from build123d import *

# Parameters (mm, degrees)
SKETCH1_R           = 1.05
BOSS_EXTRUDE1_DEPTH = 2.85
FILLET2_R           = 1
FILLET1_R           = 1


with BuildPart() as part:
    # Sketch1 → Boss-Extrude1 (new body)
    with BuildSketch(Plane.XY):
        with BuildLine():
            Line((2.236067977, 2), (15, 3.5))
            Line((15, 3.5), (15, 6))
            ThreePointArc((15, 6), (16.630733614, 7.494292047), (17.97721163, 5.739527733))
            Line((17.97721163, 5.739527733), (17.229668505, 1.5))
            Line((17.229668505, 1.5), (0, -2))
            Line((0, -2), (-17.229668505, 1.5))
            Line((-17.229668505, 1.5), (-17.97721163, 5.739527733))
            ThreePointArc((-17.97721163, 5.739527733), (-16.630733614, 7.494292047), (-15, 6))
            Line((-15, 6), (-15, 3.5))
            Line((-15, 3.5), (-2.236067977, 2))
            ThreePointArc((-2.236067977, 2), (0, 3), (2.236067977, 2))
        make_face()
        Circle(SKETCH1_R, mode=Mode.SUBTRACT)
    extrude(amount=BOSS_EXTRUDE1_DEPTH)

    # Fillet2
    fillet2_edges = [part.edges().sort_by_distance(p)[0] for p in [
        (15, 3.5, 1.425),
        (-15, 3.5, 1.425),
    ]]
    fillet(fillet2_edges, radius=FILLET2_R)

    # Fillet1
    fillet1_edges = [part.edges().sort_by_distance(p)[0] for p in [
        (15, 5.194681496, 0),
        (16.630733614, 7.494292047, 0),
        (17.603440067, 3.619763867, 0),
        (-17.603440067, 3.619763867, 0),
        (-16.630733614, 7.494292047, 0),
        (-16.630733614, 7.494292047, 2.85),
        (-8.176391715, 2.698098798, 0),
        (-17.603440067, 3.619763867, 2.85),
        (17.603440067, 3.619763867, 2.85),
        (16.630733614, 7.494292047, 2.85),
        (15, 5.194681496, 2.85),
        (-15, 5.194681496, 0),
        (-15, 5.194681496, 2.85),
        (8.176391715, 2.698098798, 0),
        (8.176391715, 2.698098798, 2.85),
        (-14.747233381, 3.724801276, 0),
        (-14.747233381, 3.724801276, 2.85),
        (14.747233381, 3.724801276, 0),
        (14.747233381, 3.724801276, 2.85),
        (-8.176391715, 2.698098798, 2.85),
    ]]
    fillet(fillet1_edges, radius=FILLET1_R)


solid = part.part
Could you check a few things on this model? Use its own coordinates, in mm. A direction names the side the tool comes from. Coordinates: 2 decimals unless noted, no trailing zeros. Loops run counter-clockwise (first coordinate to the right, second up) from the corner with the lowest first, then second, coordinate; pieces in that order, holes last. Notation, with made-up numbers: (68, 16) -> (98, 16) arc R6 cw to (98, 23) -> close; hole circle Ø2 at (46, 46.25). An arc over 180 degrees is marked (long way). Answer in a Markdown table with one row per item.
(1) If I drill on probe 1 along Y at (x, z) = (0, 1.1); probe 2 along Y at (x, z) = (-0.5, 0.45); probe 3 along X at (y, z) = (5.5, 0.6), over which ranges is the centre line in solid material (lowest first)?
Results found:
| item | result |
|---|---|
| probe 1 | y = -2 to -1.05, 1.05 to 3 |
| probe 2 | y = -1.9 to -0.92, 0.92 to 2.96 |
| probe 3 | x = -17.85 to -15.08, 15.08 to 17.85 |
(2) Will these pins go through, and if not, where does the flat tip stop? pin 1 Ø1.9 at (x, y) = (0, 0) entering from +Z; pin 2 Ø0.9 at (y, z) = (5, 1.5) entering from +X; pin 3 Ø1 at (y, z) = (3.5, 2) entering from +X.
Results found:
| item | result |
|---|---|
| pin 1 | passes through |
| pin 2 | stops at x = 17.93 |
| pin 3 | stops at x = 17.67 |
(3) Imagine slicing it at A-A (y = 0). List the corners of the cut face in (x, z) for me.
Results found:
| item | result |
|---|---|
| outline | (-9.85, 0) -> (-1.05, 0) -> (-1.05, 2.85) -> (-9.85, 2.85) -> close; (1.05, 0) -> (9.85, 0) -> (9.85, 2.85) -> (1.05, 2.85) -> close |
(4) Thinking about a two-plate mould opening in X: for faces 1 (the face through (17.267, 3.446, 0.285)), 2 (the face through (1, 0.32, 1.41)), 3 (the face through (-17.279, 3.511, 0.285)), which applies, released by +X, released by -X, zero draft, split by the parting line, or undercut?
Results found:
| item | result |
|---|---|
| face 1 | released by +X |
| face 2 | undercut |
| face 3 | released by -X |
(5) Imagine slicing it at B-B (x = 1.5). List the corners of the cut face in (y, z) for me.
Results found:
| item | result |
|---|---|
| outline | (-1.7, 0) -> (2.6, 0) -> (2.6, 2.85) -> (-1.7, 2.85) -> close |
(6) For faces 4 (the face through (15.301, 5.206, 0.285)), 5 (the face through (14.74, 3.717, 1.431)), 6 (the face through (15.301, 5.206, 2.565)), 7 (the face through (17.267, 3.446, 2.565)), which set-ups out of +Z, -Z, +X, -X, +Y, -Y let a thin tool reach every point of the face, with its end or its side?
Results found:
| item | result |
|---|---|
| face 4 | -Z, +Y |
| face 5 | +Z, -Z, +Y |
| face 6 | +Z, +Y |
| face 7 | +Z, +X, -Y |
